The listing builds one solid part. Answer for the finished solid, in the listing's coordinates (mm). A direction names the side the tool comes from. Give positions to 0.01 mm unless a question says otherwise; leave off trailing zeros. Order: outer loops, then holes, each group sorted by start corner. A loop starts at its lowest first (then second) coordinate and runs counter-clockwise, first axis right, second up. Notation, with made-up numbers: (44, 75) - (73, 75) arc R12 ccw to (73, 95) - close; hole circle Ø11 at (-20, 0). An arc over 180 degrees is marked (long way). Answer in a Markdown table with one row per item.
from build123d import *

# Parameters (mm, degrees)
F0_R     = 19
F1_DEPTH = 12.5
F2_R     = 5


with BuildPart() as f1:
    # F0 (on Top) → F1 (new body, symmetric)
    with BuildSketch(Plane.XY):
        with BuildLine():
            Line((-34.749801, 52.841643), (-21, 0))
            ThreePointArc((-21, 0), (0, -21), (21, 0))
            Line((21, 0), (34.749801, 52.841643))
            Line((34.749801, 52.841643), (32.314748, 53.410165))
            Line((32.314748, 53.410165), (25, 55.08291))
            Line((25, 55.08291), (26.631338, 53.410165))
            Line((26.631338, 53.410165), (23.264607, 48.413649))
            Line((23.264607, 48.413649), (14.595746, 15.098484))
            ThreePointArc((14.595746, 15.098484), (0, 21), (-14.595746, 15.098484))
            Line((-14.595746, 15.098484), (-23.264607, 48.413649))
            Line((-23.264607, 48.413649), (-26.631338, 53.410165))
            Line((-26.631338, 53.410165), (-25, 55.08291))
            Line((-25, 55.08291), (-32.314748, 53.410165))
            Line((-32.314748, 53.410165), (-34.749801, 52.841643))
        make_face()
        Circle(F0_R, mode=Mode.SUBTRACT)
    extrude(amount=F1_DEPTH, both=True)

    # F2
    f2_edges = [f1.edges().sort_by_distance(p)[0] for p in [
        (-14.595746, 15.098484, 0),
        (14.595746, 15.098484, 0),
    ]]
    fillet(f2_edges, radius=F2_R)


solid = f1.part
Item 1: Each of these flat-tipped pins is pushed along its axis until it touches: P1, Ø3, axis at x = 7.5, z = -3.5, coming from the -Y side; P2, Ø10, axis at y = 29.5, z = 5, coming from the +X side; P3, Ø4, axis at y = 25.5, z = -0.5, coming from the +X side; P4, Ø12, axis at x = -14.5, y = 21.5, coming from the +Z side. Where does it stop, or does it pass through?
Answer block:
| item | result |
|---|---|
| P1 | y = -20.12 |
| P2 | x = 29.98 |
| P3 | x = 28.16 |
| P4 | z = 12.5 |
Item 2: Find section B-B on z = 1.75. Write down the section's boundary in (x, y).
Answer block:
| item | result |
|---|---|
| outline | (-34.75, 52.84) - (-21, 0) arc R21 ccw to (21, 0) - (34.75, 52.84) - (32.31, 53.41) - (25, 55.08) - (26.63, 53.41) - (23.26, 48.41) - (16.4, 22.03) arc R5 cw to (9.34, 18.81) arc R21 ccw to (-9.34, 18.81) arc R5 cw to (-16.4, 22.03) - (-23.26, 48.41) - (-26.63, 53.41) - (-25, 55.08) - (-32.31, 53.41) - close; hole circle Ø38 at (0, 0) |
Item 3: Consider line 1 (Y direction, x = 0, z = 3.75); line 2 (Y direction, x = -11, z = 7); line 3 (X direction, y = 38, z = -8.5). Determine where each line is inside the solid, lowest interval first.
Answer block:
| item | result |
|---|---|
| line 1 | -21 to -19, 19 to 21 |
| line 2 | -17.89 to -15.49, 15.49 to 18.32 |
| line 3 | -30.89 to -20.55, 20.55 to 30.89 |
Item 4: Find section D-D on x = -28. Write down the section's boundary in (y, z).
Answer block:
| item | result |
|---|---|
| outline | (26.9, -12.5) - (54.4, -12.5) - (54.4, 12.5) - (26.9, 12.5) - close |
Item 5: Find section A-A on x = 0. Write down the section's boundary in (y, z), then the cut area to 4 significant figures.
Answer block:
| item | result |
|---|---|
| outline | (-21, -12.5) - (-19, -12.5) - (-19, 12.5) - (-21, 12.5) - close; (19, -12.5) - (21, -12.5) - (21, 12.5) - (19, 12.5) - close |
| area | 100.0 mm² |
Item 6: Which of the six approach directions +Z, -Z, +X, -X, +Y, -Y give full straight-line access (tool end or side, diameter ignored) to faces 1 (the face through (-25.83, 54.23, 0.18)), 2 (the face through (-28.606, 54.258, 0.175)), 3 (the face through (-19.784, 35.037, 0.175))?
Answer block:
| item | result |
|---|---|
| face 1 | +Z, -Z |
| face 2 | +Z, -Z, -X, +Y |
| face 3 | +Z, -Z, +Y |
Item 7: Find section C-C on y = 15. Write down the section's boundary in (x, z).
Answer block:
| item | result |
|---|---|
| outline | (-24.9, -12.5) - (-11.66, -12.5) - (-11.66, 12.5) - (-24.9, 12.5) - close; (11.66, -12.5) - (24.9, -12.5) - (24.9, 12.5) - (11.66, 12.5) - close |
Item 8: Determine the mould class of faces 4 (the face through (8.767, -16.856, -0.175)), 5 (the face through (-33.52, 53.13, 0.18)), 6 (the face through (-27.97, 26.79, 0.18)) for opening direction Y: pulls with the +Y half, pulls with the -Y half, needs draft (parallel to the pull), parting line crosses it, or undercut.
Answer block:
| item | result |
|---|---|
| face 4 | undercut |
| face 5 | pulls with the +Y half |
| face 6 | pulls with the -Y half |
